Autodesk Inventor part; units mm, degrees
ref_plane "YZ Plane" through (0, 0, 0) normal (1, 0, 0) x (0, 1, 0)
ref_plane "XZ Plane" through (0, 0, 0) normal (0, 1, 0) x (-1, 0, 0)
ref_plane "XY Plane" through (0, 0, 0) normal (0, 0, 1) x (1, 0, 0)
sketch "Sketch1" plane through (0, 0, 0) normal (1, 0, 0) x (0, 1, 0)
  line L0 (1.2948, 31.3833) -> (-8.7052, 31.3833)
  line L1 (-8.7052, 31.3833) -> (-8.7052, -12.6095)
  line L2 (-8.7052, -12.6095) -> (1.2948, -12.6095)
  line L3 (1.2948, -12.6095) -> (1.2948, 31.3833)
  point P0 (0, 0)
  dimension "d0" = 43.9928
  dimension "d1" = 10
extrude "Extrusion1" add sketch "Sketch1" along normal blind 38.1
sketch "Sketch2" plane through (0, 1.2948, 31.3833) normal (0, 1, 0) x (1, 0, 0)
  line L0 (38.1, 43.9928) -> (38.1, 0)
  line L1 (0, 0) -> (38.1, 0)
  line L2 (0, 43.9928) -> (38.1, 43.9928)
  point P0 (0, 31.3833)
  point P1 (19.05, 5)
  point P2 (19.05, 38.9928)
  dimension "d4" = 0
  dimension "d5" = 19.05
  dimension "d6" = 5
  dimension "d7" = 5
hole "Hole1" at (19.05, 1.2948, 26.3833) at (19.05, 1.2948, -7.6095) direction (0, -1, 0) diameter 6.7564 end through all counterbore diameter 12.7 counterbore depth 4.7752
sketch "Sketch3" plane through (0, -8.7052, -12.6095) normal (0, -1, 0) x (1, 0, 0)
  line L0 (38.1, 43.9928) -> (38.1, 0)
  line L1 (0, 43.9928) -> (0, 0)
  line L2 (0, 43.9928) -> (38.1, 43.9928)
  line L3 (0, 0) -> (38.1, 0)
  point P0 (0, 12.6095)
  point P1 (5.08, 33.8328)
  point P2 (5.08, 10.16)
  dimension "d16" = 5.08
  dimension "d24" = 10.16
  dimension "d25" = 10.16
  dimension "d26" = 5.08
hole "Hole2" at (5.08, -8.7052, 21.2233) at (5.08, -8.7052, -2.4495) direction (0, 1, 0) diameter 4.4958 end through all
properties part number "LidarV4MountShortPlate"
For this review, take the finished solid that the model builds, in its own axes (mm). A direction names the side the tool comes from. Give positions to 0.01 mm unless a question says otherwise; leave off trailing zeros. Order: outer loops, then holes, each group sorted by start corner. A loop starts at its lowest first (then second) coordinate and runs counter-clockwise, first axis right, second up.
1) For faces 1 (the face through (18.83, -1.126, 20.037)), 2 (the face through (16.201, -6.129, -5.793)), list the 3-axis set-ups (+Z, -Z, +X, -X, +Y, -Y) from which the entire face can be reached by the end or side of a thin tool; tool diameter is ignored.
2) Take a section at C-C (y = 0.75). Give the boundary of the cut face in (x, z).
3) Take a section at A-A (x = 19.05). Give the boundary of the cut face in (y, z), then the cut area to 3 significant figures.
4) Take a section at B-B (z = -7). Give the boundary of the cut face in (x, y), then the cut area to 3 significant figures.
5) Wall thickness on line 1 (X direction, y = -2.75, z = 21); line 2 (Z direction, x = 5.08, y = -2); line 3 (Z direction, x = 19.05, y = -6.85): over which ranges is each line inside the solid? List them lowest first.
6) Insertion check: pin 1 (4 mm diameter, centred on x = 5.08, z = 21.22, fed in from -Y); pin 2 (5.5 mm diameter, centred on x = 22, z = 28, fed in from +Y). Each pin has a flat end and moves straight along its axis. Give the tip position at first contact, or say it passes through.
7) The part is to be moulded in two halves that separate along X. For faces 3 (the face through (19, -8.705, 10)), 4 (the face through (20.4, -3.48, 23.1)), 5 (the face through (0, -4, 10)), say which applies: released by +X, released by -X, zero draft, split by the parting line, or undercut.
8) Take a section at D-D (x = 5.08). Give the boundary of the cut face in (y, z), then the cut area to 3 significant figures.
Derived:
1. face 1: +Y
1. face 2: +Y, -Y
2. outline: (0, -12.61) - (15.14, -12.61) arc R6.35 cw (long way) to (22.96, -12.61) - (38.1, -12.61) - (38.1, 31.38) - (22.96, 31.38) arc R6.35 cw (long way) to (15.14, 31.38) - (0, 31.38) - close; hole circle Ø4.5 at (5.08, -2.45); hole circle Ø4.5 at (5.08, 21.22)
3. outline: (-8.71, -12.61) - (-3.48, -12.61) - (-3.48, -10.99) - (-8.71, -10.99) - close; (-8.71, -4.23) - (-3.48, -4.23) - (-3.48, -1.26) - (1.29, -1.26) - (1.29, 20.03) - (-3.48, 20.03) - (-3.48, 23.01) - (-8.71, 23.01) - close; (-8.71, 29.76) - (-3.48, 29.76) - (-3.48, 31.38) - (-8.71, 31.38) - close
3. area: 261 mm2
4. outline: (0, -8.71) - (15.73, -8.71) - (15.73, -3.48) - (12.73, -3.48) - (12.73, 1.29) - (0, 1.29) - close; (22.37, -8.71) - (38.1, -8.71) - (38.1, 1.29) - (25.37, 1.29) - (25.37, -3.48) - (22.37, -3.48) - close
4. area: 286 mm2
5. line 1: x = 0 to 2.84, 7.32 to 15.68, 22.42 to 38.1
5. line 2: z = -12.61 to -4.7, -0.2 to 18.98, 23.47 to 31.38
5. line 3: z = -12.61 to -10.99, -4.23 to 23.01, 29.76 to 31.38
6. pin 1: passes through
6. pin 2: stops at y = -3.48
7. face 3: zero draft
7. face 4: undercut
7. face 5: released by -X
8. outline: (-8.71, -12.61) - (1.29, -12.61) - (1.29, -4.7) - (-8.71, -4.7) - close; (-8.71, -0.2) - (1.29, -0.2) - (1.29, 18.98) - (-8.71, 18.98) - close; (-8.71, 23.47) - (1.29, 23.47) - (1.29, 31.38) - (-8.71, 31.38) - close
8. area: 350 mm2
